```python
from build123d import *

# Parameters (mm, degrees)
SKETCH1_R           = 15
SKETCH1_R_2         = 14
BOSS_EXTRUDE1_DEPTH = 30
SKETCH2_R           = 15
SKETCH2_R_2         = 12.5
BOSS_EXTRUDE2_DEPTH = 5
SKETCH4_R           = 2.5
BOSS_EXTRUDE3_DEPTH = 23
SKETCH3_R           = 2
CUT_EXTRUDE1_DEPTH  = 35
SKETCH5_R           = 14
CUT_EXTRUDE2_DEPTH  = 53


with BuildPart() as part:
    # Sketch1 → Boss-Extrude1 (new, symmetric)
    with BuildSketch(Plane(origin=(0, 0, 0), x_dir=(0, 0, -1), z_dir=(1, 0, 0))):
        with Locations(Location((0, 0, 0), (0, 0, 180))):
            Circle(SKETCH1_R)
        with Locations(Location((0, 0, 0), (0, 0, 180))):
            Circle(SKETCH1_R_2, mode=Mode.SUBTRACT)
    extrude(amount=BOSS_EXTRUDE1_DEPTH, both=True)

    # Sketch2 → Boss-Extrude2 (add)
    with BuildSketch(Plane.ZY.offset(30)):
        Circle(SKETCH2_R)
        Circle(SKETCH2_R_2, mode=Mode.SUBTRACT)
    boss_extrude2 = extrude(amount=BOSS_EXTRUDE2_DEPTH)

    # Mirror1: Boss-Extrude2 across plane
    add(boss_extrude2.mirror(Plane(origin=(0, 0, 0), x_dir=(0, 0, 1), z_dir=(1, 0, 0))))

    # Sketch4 → Boss-Extrude3 (add)
    with BuildSketch(Plane(origin=(0, 0, 0), x_dir=(1, 0, 0), z_dir=(0, 1, 0))):
        with Locations(Location((0, 0, 0), (0, 0, 90))):
            Circle(SKETCH4_R)
    extrude(amount=BOSS_EXTRUDE3_DEPTH)

    # Sketch3 → Cut-Extrude1 (cut)
    with BuildSketch(Plane(origin=(0, 0, 0), x_dir=(1, 0, 0), z_dir=(0, 1, 0))):
        with Locations(Location((0, 0, 0), (0, 0, 270))):
            Circle(SKETCH3_R)
    extrude(amount=CUT_EXTRUDE1_DEPTH, mode=Mode.SUBTRACT)

    # Sketch5 → Cut-Extrude2 (cut)
    with BuildSketch(Plane(origin=(-30, 0, 0), x_dir=(0, 0, -1), z_dir=(1, 0, 0))):
        Circle(SKETCH5_R)
    extrude(amount=CUT_EXTRUDE2_DEPTH, mode=Mode.SUBTRACT)


solid = part.part
```
Source: CAD feature listing. Evaluate the final solid. Frame: model axes, mm. A direction names the side the tool comes from. Give positions to 0.01 mm unless a question says otherwise; leave off trailing zeros. Loops run counter-clockwise (first coordinate to the right, second up) from the corner with the lowest first, then second, coordinate; pieces in that order, holes last. Notation, with made-up numbers: (40.25, -6) -> (51.25, -6) arc R33 ccw to (51.25, 33) -> close; hole circle Ø2 at (-9.5, 54). An arc over 180 degrees is marked (long way). Put each result on its own line as item: value. Start each with the question number.
1) Material intervals for probe 1 along Y at (x, z) = (-33.65, 0); probe 2 along Y at (x, z) = (-17, 0); probe 3 along Z at (x, y) = (19.5, 0.5), sorted ascending.
2) Draft query along Z for faces 4 (the face through (-0.49, -14.643, -3.252)), 5 (the face through (32.465, 3.755, 11.923)), 6 (the face through (35, 12.3, -3.4)). Return one class per face: released by +Z, released by -Z, zero draft, split by the parting line, or undercut.
3) Reachability of faces 1 (the face through (-2, 23, 1)), 2 (the face through (-30, 11.5, -5.3)), 3 (the face through (2.44, 18.83, 0.54)) from +Z, -Z, +X, -X, +Y, -Y: full face, straight path, thin tool, end or side. Return the list, or none.
4) Cut plane A-A (y = 0). Return loops of the section in (x, z).
5) Cut plane D-D (x = 0). Return loops of the section in (y, z).
6) Contact query for flat-ended pins moving along their axis: P1, Ø4, axis at x = -24.5, z = 6, coming from the +Y side; P2, Ø2, axis at x = -14.5, y = -4, coming from the -Z side; P3, Ø5, axis at x = 7.5, z = -10.5, coming from the +Y side. Output: stop coordinate, or through.
7) Cut plane C-C (z = 10.5). Return loops of the section in (x, y).
8) Cut plane B-B (z = 0). Return loops of the section in (x, y).
Results are:
1. probe 1: y = -15 to -12.5, 12.5 to 15
1. probe 2: y = -15 to -14, 14 to 15
1. probe 3: z = -14.99 to -13.99, 13.99 to 14.99
2. face 4: split by the parting line
2. face 5: undercut
2. face 6: zero draft
3. face 1: +Z, -Z, +X, -X, +Y
3. face 2: none
3. face 3: +Y
4. outline: (-35, -15) -> (35, -15) -> (35, -12.5) -> (30, -12.5) -> (30, -14) -> (-30, -14) -> (-30, -12.5) -> (-35, -12.5) -> close; (-35, 12.5) -> (-30, 12.5) -> (-30, 14) -> (30, 14) -> (30, 12.5) -> (35, 12.5) -> (35, 15) -> (-35, 15) -> close
5. outline: (13.86, -2) arc R14 cw (long way) to (13.86, 2) -> (23, 2) -> (23, 2.5) -> (14.79, 2.5) arc R15 ccw (long way) to (14.79, -2.5) -> (23, -2.5) -> (23, -2) -> close
6. P1: stops at y = 14.46
6. P2: stops at z = -14.7
6. P3: stops at y = 12.69
7. outline: (-35, -10.71) -> (35, -10.71) -> (35, -6.78) -> (30, -6.78) -> (30, -9.26) -> (-30, -9.26) -> (-30, -6.78) -> (-35, -6.78) -> close; (-35, 6.78) -> (-30, 6.78) -> (-30, 9.26) -> (30, 9.26) -> (30, 6.78) -> (35, 6.78) -> (35, 10.71) -> (-35, 10.71) -> close
8. outline: (-35, -15) -> (35, -15) -> (35, -12.5) -> (30, -12.5) -> (30, -14) -> (-30, -14) -> (-30, -12.5) -> (-35, -12.5) -> close; (-35, 12.5) -> (-30, 12.5) -> (-30, 14) -> (-2, 14) -> (-2, 23) -> (-2.5, 23) -> (-2.5, 15) -> (-35, 15) -> close; (2, 14) -> (30, 14) -> (30, 12.5) -> (35, 12.5) -> (35, 15) -> (2.5, 15) -> (2.5, 23) -> (2, 23) -> close
